Source: three-view drawing plus pictorial views. Frame: mm from the lowest corner of the part. A direction names the side the tool comes from. Give positions to 0.01 mm unless a question says otherwise; leave off trailing zeros. Write each loop counter-clockwise with the first axis right and the second up, starting at its lowest first coordinate (ties: lowest second). Pieces come first, ordered by that corner, then holes.
Q1. Line query: L1, parallel to Z at x = 90.5, y = 9. Output: solid intervals per line, ascending.
Q2. Cut plane A-A on y = 5. Return the cut outline in (x, z).
Q3. Reachability of the marked faces 1 and 2 from +Z, -Z, +X, -X, +Y, -Y: full face, straight path, thin tool, end or side. Return the list, or none.
Q4. Cut plane C-C on x = 48.5. Return the cut outline in (y, z).
Q5. Cut plane B-B on z = 11. Return the cut outline in (x, y).
Q6. Draft query along Z for the marked faces 3, 4 and 5. Return one class per face: pulls with the +Z half, pulls with the -Z half, needs draft (parallel to the pull), parting line crosses it, or undercut.
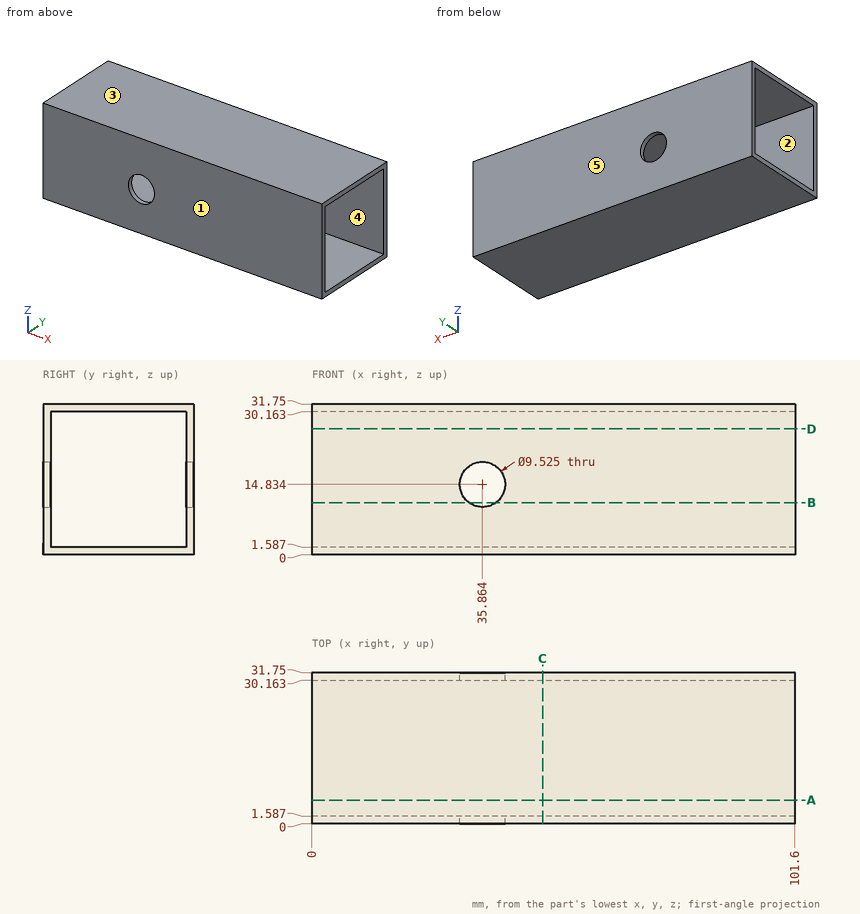
Data:
1. L1: z = 0 to 1.59, 30.16 to 31.75
2. outline: (0, 0) - (101.6, 0) - (101.6, 1.59) - (0, 1.59) - close; (0, 30.16) - (101.6, 30.16) - (101.6, 31.75) - (0, 31.75) - close
3. face 1: +Z, -Z, +X, -X, -Y
3. face 2: +X, -X
4. outline: (0, 0) - (31.75, 0) - (31.75, 31.75) - (0, 31.75) - close; hole (1.59, 1.59) - (30.16, 1.59) - (30.16, 30.16) - (1.59, 30.16) - close
5. outline: (0, 0) - (33.04, 0) - (33.04, 1.59) - (0, 1.59) - close; (0, 30.16) - (33.04, 30.16) - (33.04, 31.75) - (0, 31.75) - close; (38.69, 0) - (101.6, 0) - (101.6, 1.59) - (38.69, 1.59) - close; (38.69, 30.16) - (101.6, 30.16) - (101.6, 31.75) - (38.69, 31.75) - close
6. face 3: pulls with the +Z half
6. face 4: undercut
6. face 5: needs draft
